Input: part model. Units: mm. Frame: model coordinates. Face numbers are marked on the shaded views. A direction names the side the tool comes from. Round coordinates to 2 decimals unless told otherwise and drop trailing zeros. Loops run counter-clockwise (first coordinate to the right, second up) from the corner with the lowest first, then second, coordinate; pieces in that order, holes last. Notation, with made-up numbers: M 23,-16 L 59,-16 A18 ccw 59,9 Z; hole C 85,83.25 d1. An arc over 180 degrees is marked long. Put each result on its own line as item: value. Start each with the question number.
1) Section C-C on y = 2.75. Output: boundary loops of the cut face in (x, z).
2) Draft query along Z for the marked faces 5, 6 and 7. Return one class per face: +Z half, -Z half, draft (parallel to the pull), parting line (faces both ways), or undercut.
3) Pin query (flat end, axial travel): pin 1 (0.6 mm diameter, centred on x = -54.5, z = -2.5, fed in from +Y); pin 2 (6 mm diameter, centred on x = -56.5, z = -3.5, fed in from -Y); pin 3 (1.5 mm diameter, centred on x = -54, z = -17.5, fed in from -Y). Return the tip coordinate at first contact, or that it passes through.
4) Section A-A on x = -51.25. Output: boundary loops of the cut face in (y, z).
5) Reachability of the marked faces 1, 2, 3 and 4 from +Z, -Z, +X, -X, +Y, -Y: full face, straight path, thin tool, end or side. Return the list, or none.
6) Section D-D on z = -13.25. State how many separate pieces and enclosed holes the cut face has, plus the area to 3 significant figures.
7) Line query: probe 1 along Z at (x, y) = (-57, 4.75); probe 2 along Z at (x, y) = (-59, 3.75); probe 3 along Y at (x, z) = (-53.5, -13.25). Output: solid intervals per line, ascending.
from build123d import *

# Parameters (mm, degrees)
BOSS_EXTRUDE1_DEPTH = 5
SKETCH2_W           = 11
SKETCH2_H           = 6
BOSS_EXTRUDE2_DEPTH = 8
SKETCH3_W           = 9
SKETCH3_H           = 2
CUT_EXTRUDE1_DEPTH  = 2
SKETCH5_W           = 9
SKETCH5_H           = 3
CUT_EXTRUDE2_DEPTH  = 2
SKETCH7_W           = 11
SKETCH7_H           = 7
BOSS_EXTRUDE3_DEPTH = 8
SKETCH8_W           = 7
SKETCH8_H           = 2
BOSS_EXTRUDE4_DEPTH = 1
SKETCH9_W           = 2
SKETCH9_H           = 1
CUT_EXTRUDE3_DEPTH  = 1
SKETCH10_W          = 7
SKETCH10_H          = 3
BOSS_EXTRUDE5_DEPTH = 1
BOSS_EXTRUDE6_DEPTH = 7
BOSS_EXTRUDE7_DEPTH = 5
SKETCH14_W          = 0.5
SKETCH14_H          = 2
CUT_EXTRUDE4_DEPTH  = 1
SKETCH15_W          = 7
SKETCH15_H          = 3
CUT_EXTRUDE5_DEPTH  = 8
SKETCH16_R          = 0.25
CUT_EXTRUDE10_DEPTH = 10
FILLET1_R           = 0.5


with BuildPart() as part:
    # Sketch1 → Boss-Extrude1 (new body)
    with BuildSketch(Plane.XY):
        Polygon((-53.574922408, 6), (-50.824922408, 6), (-50.824922408, 0), (-61.824922408, 0), (-61.824922408, 6), (-59.074922408, 6), (-59.074922408, 4), (-58.574922408, 4), (-58.574922408, 6), (-58.074922408, 6), (-58.074922408, 4), (-57.574922408, 4), (-57.574922408, 6), (-57.074922408, 6), (-57.074922408, 4), (-56.574922408, 4), (-56.574922408, 6), (-56.074922408, 6), (-56.074922408, 4), (-55.574922408, 4), (-55.574922408, 6), (-55.074922408, 6), (-55.074922408, 4), (-54.574922408, 4), (-54.574922408, 6), (-54.074922408, 6), (-54.074922408, 4), (-53.574922408, 4), align=None)
    extrude(amount=-BOSS_EXTRUDE1_DEPTH)

    # Sketch2 → Boss-Extrude2 (add)
    with BuildSketch(Plane(origin=(0, 0, -5), x_dir=(-1, 0, 0), z_dir=(0, 0, -1))):
        with Locations((56.324922408, 3)):
            Rectangle(SKETCH2_W, SKETCH2_H)
    extrude(amount=BOSS_EXTRUDE2_DEPTH)

    # Sketch3 → Cut-Extrude1 (cut)
    with BuildSketch(Plane(origin=(0, 6, 0), x_dir=(1, 0, 0), z_dir=(0, 1, 0))):
        with Locations((-56.324922408, 7)):
            Rectangle(SKETCH3_W, SKETCH3_H)
    extrude(amount=-CUT_EXTRUDE1_DEPTH, mode=Mode.SUBTRACT)

    # Sketch5 → Cut-Extrude2 (cut)
    with BuildSketch(Plane(origin=(0, 6, 0), x_dir=(1, 0, 0), z_dir=(0, 1, 0))):
        with Locations((-56.324922408, 10.5)):
            Rectangle(SKETCH5_W, SKETCH5_H)
    extrude(amount=-CUT_EXTRUDE2_DEPTH, mode=Mode.SUBTRACT)

    # Sketch7 → Boss-Extrude3 (add)
    with BuildSketch(Plane(origin=(0, 0, -13), x_dir=(-1, 0, 0), z_dir=(0, 0, -1))):
        with Locations((56.324922408, 3.5)):
            Rectangle(SKETCH7_W, SKETCH7_H)
    extrude(amount=BOSS_EXTRUDE3_DEPTH)

    # Sketch8 → Boss-Extrude4 (add)
    with BuildSketch(Plane.XY):
        with Locations((-56.324922408, 0)):
            Rectangle(SKETCH8_W, SKETCH8_H)
    extrude(amount=BOSS_EXTRUDE4_DEPTH)

    # Sketch9 → Cut-Extrude3 (cut)
    with BuildSketch(Plane.XY):
        with Locations((-60.824922408, 0.5)):
            Rectangle(SKETCH9_W, SKETCH9_H)
        with Locations((-51.824922408, 0.5)):
            Rectangle(SKETCH9_W, SKETCH9_H)
    extrude(amount=-CUT_EXTRUDE3_DEPTH, mode=Mode.SUBTRACT)

    # Sketch10 → Boss-Extrude5 (add)
    with BuildSketch(Plane.XZ):
        with Locations((-56.324922408, -1.5)):
            Rectangle(SKETCH10_W, SKETCH10_H)
    extrude(amount=BOSS_EXTRUDE5_DEPTH)

    # Sketch12 → Boss-Extrude6 (add)
    with BuildSketch(Plane(origin=(-52.824922408, 0, 0), x_dir=(0, 0, -1), z_dir=(1, 0, 0))):
        Polygon((3, 0), (5.992424207, -0.484369133), (5.992424207, -2.095529726), (4.896502139, -1.339612629), (3, -1), align=None)
    extrude(amount=-BOSS_EXTRUDE6_DEPTH)

    # Sketch13 → Boss-Extrude7 (add)
    with BuildSketch(Plane(origin=(-53.824922408, 0, 0), x_dir=(0, 0, -1), z_dir=(1, 0, 0))):
        with BuildLine():
            Line((14.148954215, -2.461888554), (14.148954215, -2.839825861))
            ThreePointArc((14.148954215, -2.839825861), (14.071635021, -3.040856353), (13.87953249, -3.138263407))
            add(Edge.make_bspline(
                [(5.992424207, -2.095529726), (8.29118563, -2.416616876), (10.932584268, -1.908869196), (13.449456914, -2.990370177), (13.696503578, -3.157016773), (13.87953249, -3.138263407)],
                knots=[0, 0, 0, 0, 0.841667249, 0.882833834, 0.948247019, 0.948247019, 0.948247019, 0.948247019], degree=3))
            Line((5.992424207, -2.095529726), (5.992424207, -0.484369133))
            add(Edge.make_bspline(
                [(5.992424207, -0.484369133), (8.707741723, -0.750205277), (11.359938613, -1.314908717), (13.943929605, -2.177319274)],
                knots=[0, 0, 0, 0, 0.957734947, 0.957734947, 0.957734947, 0.957734947], degree=3))
            ThreePointArc((13.943929605, -2.177319274), (14.092359861, -2.28652125), (14.148954215, -2.461888554))
        make_face()
    extrude(amount=-BOSS_EXTRUDE7_DEPTH)

    # Sketch14 → Cut-Extrude4 (cut)
    with BuildSketch(Plane(origin=(0, 4, 0), x_dir=(1, 0, 0), z_dir=(0, 1, 0))):
        with Locations((-53.824922408, 2.5)):
            Rectangle(SKETCH14_W, SKETCH14_H)
        with Locations((-54.824922408, 2.5)):
            Rectangle(SKETCH14_W, SKETCH14_H)
        with Locations((-55.824922408, 2.5)):
            Rectangle(SKETCH14_W, SKETCH14_H)
        with Locations((-56.824922408, 2.5)):
            Rectangle(SKETCH14_W, SKETCH14_H)
        with Locations((-57.824922408, 2.5)):
            Rectangle(SKETCH14_W, SKETCH14_H)
        with Locations((-58.824922408, 2.5)):
            Rectangle(SKETCH14_W, SKETCH14_H)
    extrude(amount=-CUT_EXTRUDE4_DEPTH, mode=Mode.SUBTRACT)

    # Sketch15 → Cut-Extrude5 (cut)
    with BuildSketch(Plane(origin=(0, 0, -21), x_dir=(-1, 0, 0), z_dir=(0, 0, -1))):
        with Locations((56.324922408, 3.5)):
            Rectangle(SKETCH15_W, SKETCH15_H)
    extrude(amount=-CUT_EXTRUDE5_DEPTH, mode=Mode.SUBTRACT)

    # Sketch16 → Cut-Extrude10 (cut)
    with BuildSketch(Plane(origin=(0, 0, -13), x_dir=(-1, 0, 0), z_dir=(0, 0, -1))):
        with Locations((53.824922408, 3.25)):
            Circle(SKETCH16_R)
        with Locations((54.824922408, 3.25)):
            Circle(SKETCH16_R)
        with Locations((55.824922408, 3.25)):
            Circle(SKETCH16_R)
        with Locations((56.824922408, 3.25)):
            Circle(SKETCH16_R)
        with Locations((57.824922408, 3.25)):
            Circle(SKETCH16_R)
        with Locations((58.824922408, 3.25)):
            Circle(SKETCH16_R)
    extrude(amount=-CUT_EXTRUDE10_DEPTH, mode=Mode.SUBTRACT)

    # Fillet1
    fillet1_edges = [part.edges().sort_by_distance(p)[0] for p in [
        (-60.449922408, 6, 0),
        (-58.324922408, 6, 0),
        (-57.324922408, 6, 0),
        (-56.324922408, 6, 0),
        (-55.324922408, 6, 0),
        (-54.324922408, 6, 0),
        (-52.199922408, 6, 0),
    ]]
    fillet(fillet1_edges, radius=FILLET1_R)


solid = part.part
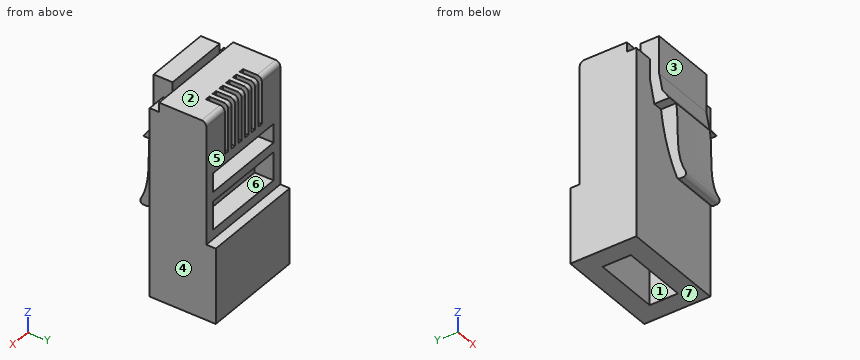
Geometry results:
1. outline: M -61.82,-21 L -59.82,-21 L -59.82,-13 L -52.82,-13 L -52.82,-21 L -50.82,-21 L -50.82,0 L -61.82,0 Z
2. face 5: draft
2. face 6: undercut
2. face 7: -Z half
3. pin 1: stops at y = 6
3. pin 2: stops at y = -2.15
3. pin 3: stops at y = 0
4. outline: M 0,-21 L 7,-21 L 7,-13 L 6,-13 L 6,-0.5 A0.5 ccw 5.5,0 L 1,0 L 1,-1 L 0,-1 Z
5. face 1: -Z
5. face 2: +Z, +X, -X, +Y
5. face 3: +Z, +X, -X, -Y
5. face 4: +Z, -Z, +X, +Y, -Y
6. separate pieces: 2
6. enclosed holes: 1
6. area: 60.8 mm²
7. probe 1: z = -13 to -12, -9 to -8, -6 to -5
7. probe 2: z = -13 to -3.5, -1.5 to 0
7. probe 3: y = 0 to 2, 5 to 7
